```python
from build123d import *

# Parameters (mm, degrees)
SKETCH1_W           = 40
SKETCH1_H           = 40
BOSS_EXTRUDE1_DEPTH = 3
SKETCH2_R           = 3
CUT_EXTRUDE1_DEPTH  = 3
SKETCH3_W           = 5
SKETCH3_H           = 3
CUT_EXTRUDE2_DEPTH  = 10
SKETCH4_W           = 3
SKETCH4_H           = 5
CUT_EXTRUDE3_DEPTH  = 3


with BuildPart() as part:
    # Sketch1 → Boss-Extrude1 (new body)
    with BuildSketch(Plane(origin=(0, 0, 0), x_dir=(1, 0, 0), z_dir=(0, 1, 0))):
        Rectangle(SKETCH1_W, SKETCH1_H)
    extrude(amount=BOSS_EXTRUDE1_DEPTH)

    # Sketch2 → Cut-Extrude1 (cut)
    with BuildSketch(Plane(origin=(0, 3, 0), x_dir=(1, 0, 0), z_dir=(0, 1, 0))):
        with Locations(Location((0, 0, 0), (0, 0, 270))):
            Circle(SKETCH2_R)
    extrude(amount=-CUT_EXTRUDE1_DEPTH, mode=Mode.SUBTRACT)

    # Sketch3 → Cut-Extrude2 (cut)
    with BuildSketch(Plane.XZ):
        with Locations((12.5, -18.5)):
            Rectangle(SKETCH3_W, SKETCH3_H)
        with Locations((-12.5, -18.5)):
            Rectangle(SKETCH3_W, SKETCH3_H)
    extrude(amount=-CUT_EXTRUDE2_DEPTH, mode=Mode.SUBTRACT)

    # Sketch4 → Cut-Extrude3 (cut)
    with BuildSketch(Plane.XZ):
        with Locations((18.5, 12.5)):
            Rectangle(SKETCH4_W, SKETCH4_H)
        with Locations((18.5, -9.5)):
            Rectangle(SKETCH4_W, SKETCH4_H)
        with Locations((-18.5, -9.5)):
            Rectangle(SKETCH4_W, SKETCH4_H)
        with Locations((-18.5, 12.5)):
            Rectangle(SKETCH4_W, SKETCH4_H)
    extrude(amount=-CUT_EXTRUDE3_DEPTH, mode=Mode.SUBTRACT)


solid = part.part
```
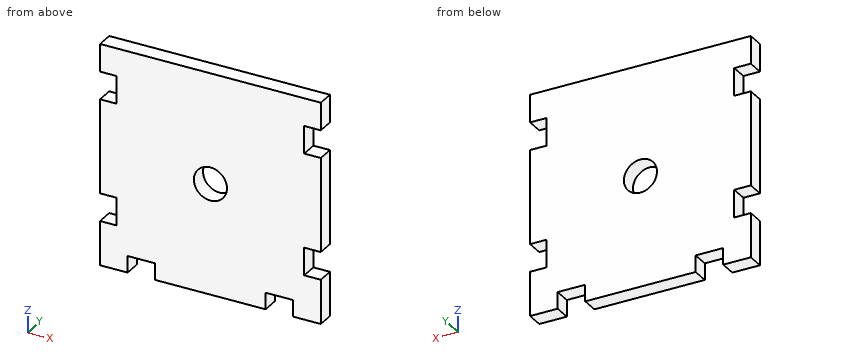
Design review of the part built by this model. Coordinates are the model's own, in mm. Round coordinates to 2 decimals unless told otherwise and drop trailing zeros. Order: outer loops, then holes, each group sorted by start corner. A loop starts at its lowest first (then second) coordinate and runs counter-clockwise, first axis right, second up. Notation, with made-up numbers: M 40.25,81 L 57.25,81 A28 ccw 57.25,115 Z; hole C 31.25,6.5 d5. An arc over 180 degrees is marked long. Put each result on its own line as item: value.
Q1. Consider section B-B (x = 0). State the section outline as (y, z) points.
Reported:
outline: M 0,-20 L 3,-20 L 3,-3 L 0,-3 Z; M 0,3 L 3,3 L 3,20 L 0,20 Z
Q2. Consider section D-D (x = 14). State the section outline as (y, z) points, and give its area (3 significant figures).
Reported:
outline: M 0,-17 L 3,-17 L 3,20 L 0,20 Z
area: 111 mm²
Q3. Consider section A-A (z = 0). State the section outline as (x, y) points.
Reported:
outline: M -20,0 L -3,0 L -3,3 L -20,3 Z; M 3,0 L 20,0 L 20,3 L 3,3 Z
Q4. Insertion check: pin 1 Ø1.5 at (y, z) = (2, 12.5) entering from +X; pin 2 Ø0.9 at (y, z) = (1.5, -9) entering from -X. Each pin has a flat end and moves straight along its axis. Give the tip position at first contact, or say it passes through.
Reported:
pin 1: x = 17
pin 2: x = -17
Q5. To check wall thickness, follow line 1 (X direction, y = 2.6, z = -17.5); line 2 (X direction, y = 1.8, z = 0); line 3 (Z direction, x = 12, y = 2.2). State the ranges of each line that lie inside material, in increasing order.
Reported:
line 1: -20 to -15, -10 to 10, 15 to 20
line 2: -20 to -3, 3 to 20
line 3: -17 to 20
